Check sheet for the modelled part. Datum: model origin and axes. Units: mm. A direction names the side the tool comes from. Round coordinates to 2 decimals unless told otherwise and drop trailing zeros. Order: outer loops, then holes, each group sorted by start corner. A loop starts at its lowest first (then second) coordinate and runs counter-clockwise, first axis right, second up.
from build123d import *

# Parameters (mm, degrees)
F0_W     = 1
F0_H     = 54
F0_W_2   = 1.75
F0_H_2   = 35
F0_R     = 3
F0_R_2   = 1.25
F1_DEPTH = 2
F2_DEPTH = 20
F3_DEPTH = 13
F4_DEPTH = 10
F5_DEPTH = 20
F6_DEPTH = 13


# Not quite as in the source:
# - a feature names something its author has since deleted; it is built from what else it names


with BuildPart() as f1:
    # F0 (on Top) → F1 (new body)
    with BuildSketch(Plane.XY):
        Polygon((10.25, 0), (-142.25, 0), (-142.25, -10.5), (-141.25, -10.5), (-141.25, -1), (10.25, -1), align=None)
        Polygon((46, 0), (10.25, 0), (10.25, -1), (10.25, -2), (44.25, -2), (44.25, -11.5), (46, -11.5), align=None)
        with Locations((-141.75, -37.5)):
            Rectangle(F0_W, F0_H)
        Polygon((10.25, -2), (10.25, -1), (-141.25, -1), (-141.25, -10.5), (-140.25, -10.5), (-140.25, -2), align=None)
        Polygon((-141.25, -64.5), (-142.25, -64.5), (-142.25, -94.5), (10.25, -94.5), (10.25, -93.5), (-141.25, -93.5), align=None)
        with Locations((-140.75, -37.5)):
            Rectangle(F0_W, F0_H)
        with Locations((45.125, -29)):
            Rectangle(F0_W_2, F0_H_2)
        Polygon((44.25, -2), (10.25, -2), (-140.25, -2), (-140.25, -10.5), (-140.25, -64.5), (-140.25, -92.5), (10.25, -92.5), (44.25, -92.5), (44.25, -46.5), (44.25, -11.5), align=None)
        with Locations((-135, -87.25)):
            Circle(F0_R, mode=Mode.SUBTRACT)
        with Locations((-75, -87.25)):
            Circle(F0_R, mode=Mode.SUBTRACT)
        with Locations((0, -87.25)):
            Circle(F0_R, mode=Mode.SUBTRACT)
        with Locations((39, -87.25)):
            Circle(F0_R, mode=Mode.SUBTRACT)
        with Locations((-135, -7.25)):
            Circle(F0_R, mode=Mode.SUBTRACT)
        with Locations((-75, -7.25)):
            Circle(F0_R, mode=Mode.SUBTRACT)
        with Locations((0, -7.25)):
            Circle(F0_R, mode=Mode.SUBTRACT)
        with Locations((39, -7.25)):
            Circle(F0_R, mode=Mode.SUBTRACT)
        Polygon((-140.25, -64.5), (-141.25, -64.5), (-141.25, -93.5), (10.25, -93.5), (10.25, -92.5), (-140.25, -92.5), align=None)
        Polygon((46, -94.5), (46, -46.5), (44.25, -46.5), (44.25, -92.5), (10.25, -92.5), (10.25, -93.5), (10.25, -94.5), align=None)
        with Locations((-135, -87.25)):
            Circle(F0_R)
        with Locations((-135, -87.25)):
            Circle(F0_R_2, mode=Mode.SUBTRACT)
        with Locations((-135, -7.25)):
            Circle(F0_R)
        with Locations((-135, -7.25)):
            Circle(F0_R_2, mode=Mode.SUBTRACT)
        with Locations((-75, -87.25)):
            Circle(F0_R)
        with Locations((-75, -87.25)):
            Circle(F0_R_2, mode=Mode.SUBTRACT)
        with Locations((-75, -7.25)):
            Circle(F0_R)
        with Locations((-75, -7.25)):
            Circle(F0_R_2, mode=Mode.SUBTRACT)
        with Locations((0, -7.25)):
            Circle(F0_R)
        with Locations((0, -7.25)):
            Circle(F0_R_2, mode=Mode.SUBTRACT)
        with Locations((0, -87.25)):
            Circle(F0_R)
        with Locations((0, -87.25)):
            Circle(F0_R_2, mode=Mode.SUBTRACT)
        with Locations((39, -87.25)):
            Circle(F0_R)
        with Locations((39, -87.25)):
            Circle(F0_R_2, mode=Mode.SUBTRACT)
        with Locations((39, -7.25)):
            Circle(F0_R)
        with Locations((39, -7.25)):
            Circle(F0_R_2, mode=Mode.SUBTRACT)
        with Locations((-135, -87.25)):
            Circle(F0_R_2)
        with Locations((-75, -87.25)):
            Circle(F0_R_2)
        with Locations((0, -87.25)):
            Circle(F0_R_2)
        with Locations((39, -87.25)):
            Circle(F0_R_2)
        with Locations((-135, -7.25)):
            Circle(F0_R_2)
        with Locations((-75, -7.25)):
            Circle(F0_R_2)
        with Locations((0, -7.25)):
            Circle(F0_R_2)
        with Locations((39, -7.25)):
            Circle(F0_R_2)
    extrude(amount=-F1_DEPTH)

    # F0 (on Top) → F2 (join)
    with BuildSketch(Plane.XY):
        Polygon((10.25, 0), (-142.25, 0), (-142.25, -10.5), (-141.25, -10.5), (-141.25, -1), (10.25, -1), align=None)
        Polygon((46, 0), (10.25, 0), (10.25, -1), (10.25, -2), (44.25, -2), (44.25, -11.5), (46, -11.5), align=None)
        Polygon((46, -94.5), (46, -46.5), (44.25, -46.5), (44.25, -92.5), (10.25, -92.5), (10.25, -93.5), (10.25, -94.5), align=None)
        Polygon((-141.25, -64.5), (-142.25, -64.5), (-142.25, -94.5), (10.25, -94.5), (10.25, -93.5), (-141.25, -93.5), align=None)
    extrude(amount=F2_DEPTH)

    # F0 (on Top) → F3 (join)
    with BuildSketch(Plane.XY):
        Polygon((10.25, -2), (10.25, -1), (-141.25, -1), (-141.25, -10.5), (-140.25, -10.5), (-140.25, -2), align=None)
        Polygon((-140.25, -64.5), (-141.25, -64.5), (-141.25, -93.5), (10.25, -93.5), (10.25, -92.5), (-140.25, -92.5), align=None)
    extrude(amount=F3_DEPTH)

    # F0 (on Top) → F4 (join)
    with BuildSketch(Plane.XY):
        with Locations((-140.75, -37.5)):
            Rectangle(F0_W, F0_H)
        with Locations((-141.75, -37.5)):
            Rectangle(F0_W, F0_H)
        with Locations((45.125, -29)):
            Rectangle(F0_W_2, F0_H_2)
    extrude(amount=F4_DEPTH)

    # F0 (on Top) → F5 (join)
    with BuildSketch(Plane.XY):
        with Locations((-135, -7.25)):
            Circle(F0_R_2)
        with Locations((-75, -7.25)):
            Circle(F0_R_2)
        with Locations((0, -7.25)):
            Circle(F0_R_2)
        with Locations((39, -7.25)):
            Circle(F0_R_2)
        with Locations((39, -87.25)):
            Circle(F0_R_2)
        with Locations((0, -87.25)):
            Circle(F0_R_2)
        with Locations((-75, -87.25)):
            Circle(F0_R_2)
        with Locations((-135, -87.25)):
            Circle(F0_R_2)
    extrude(amount=F5_DEPTH)

    # F0 (on Top) → F6 (join)
    with BuildSketch(Plane.XY):
        with Locations((-135, -7.25)):
            Circle(F0_R)
        with Locations((-135, -7.25)):
            Circle(F0_R_2, mode=Mode.SUBTRACT)
        with Locations((-75, -7.25)):
            Circle(F0_R)
        with Locations((-75, -7.25)):
            Circle(F0_R_2, mode=Mode.SUBTRACT)
        with Locations((0, -7.25)):
            Circle(F0_R)
        with Locations((0, -7.25)):
            Circle(F0_R_2, mode=Mode.SUBTRACT)
        with Locations((39, -7.25)):
            Circle(F0_R)
        with Locations((39, -7.25)):
            Circle(F0_R_2, mode=Mode.SUBTRACT)
        with Locations((-135, -87.25)):
            Circle(F0_R)
        with Locations((-135, -87.25)):
            Circle(F0_R_2, mode=Mode.SUBTRACT)
        with Locations((-75, -87.25)):
            Circle(F0_R)
        with Locations((-75, -87.25)):
            Circle(F0_R_2, mode=Mode.SUBTRACT)
        with Locations((0, -87.25)):
            Circle(F0_R)
        with Locations((0, -87.25)):
            Circle(F0_R_2, mode=Mode.SUBTRACT)
        with Locations((39, -87.25)):
            Circle(F0_R)
        with Locations((39, -87.25)):
            Circle(F0_R_2, mode=Mode.SUBTRACT)
    extrude(amount=F6_DEPTH)


solid = f1.part
1) Sectioned sample at D-D on y = -14. Record the cut outline in (x, z), and give its area (3 significant figures).
2) Sectioned sample at C-C on x = -119.5. Record the cut outline in (y, z), and give its area (3 significant figures).
3) Set-up check for faces 1 (the face through (46, -48, 9)), 2 (the face through (-47, -92.5, 8)): record each of +Z, -Z, +X, -X, +Y, -Y from which the full face is reachable in a straight line by a thin tool's end or side.
4) Draft check along Y on faces 3 (the face through (-49, -94.5, 9)), 4 (the face through (-47, 0, 9)), 5 (the face through (-142.25, -48, 6)), 6 (the face through (44.25, -47, 10)). Enter one of: pulls with the +Y half, pulls with the -Y half, needs draft (parallel to the pull), parting line crosses it, or undercut.
5) Gauge pin test, flat ends, axial feed: pin 1 (0.6 mm diameter, centred on x = -141, z = 15.5, fed in from +Y); pin 2 (6 mm diameter, centred on y = -47.5, z = 17.5, fed in from -X); pin 3 (12 mm diameter, centred on x = 1.5, y = -74.5, fed in from +Z); pin 4 (1.6 mm diameter, centred on x = -141, y = -35.5, fed in from +Z). Record the tip position at first contact, or that the pin passes through.
6) Sectioned sample at B-B on y = -82. Record the cut outline in (x, z).
7) Sectioned sample at A-A on z = 5.5. Count the separate pieces of the cut face and the enclosed holes in it, and give its area (3 significant figures).
8) Scan lines: line 1 (X direction, y = -35.5, z = 1); line 2 (Y direction, x = -66.5, z = 7.25); line 3 (X direction, y = -69, z = 14.75). Record each from-to range of solid material in increasing order.
Values found:
1. outline: (-142.25, -2) - (46, -2) - (46, 10) - (44.25, 10) - (44.25, 0) - (-140.25, 0) - (-140.25, 10) - (-142.25, 10) - close
1. area: 414 mm2
2. outline: (-94.5, -2) - (0, -2) - (0, 20) - (-1, 20) - (-1, 13) - (-2, 13) - (-2, 0) - (-92.5, 0) - (-92.5, 13) - (-93.5, 13) - (-93.5, 20) - (-94.5, 20) - close
2. area: 255 mm2
3. face 1: +Z, -Z, +X, +Y, -Y
3. face 2: +Z
4. face 3: pulls with the -Y half
4. face 4: pulls with the +Y half
4. face 5: needs draft
4. face 6: undercut
5. pin 1: stops at y = 0
5. pin 2: stops at x = 44.25
5. pin 3: stops at z = 0
5. pin 4: stops at z = 10
6. outline: (-142.25, -2) - (46, -2) - (46, 20) - (44.25, 20) - (44.25, 0) - (-140.25, 0) - (-140.25, 13) - (-141.25, 13) - (-141.25, 20) - (-142.25, 20) - close
7. separate pieces: 9
7. enclosed holes: 1
7. area: 1,320 mm2
8. line 1: x = -142.25 to -140.25, 44.25 to 46
8. line 2: y = -94.5 to -92.5, -2 to 0
8. line 3: x = -142.25 to -141.25, 44.25 to 46
